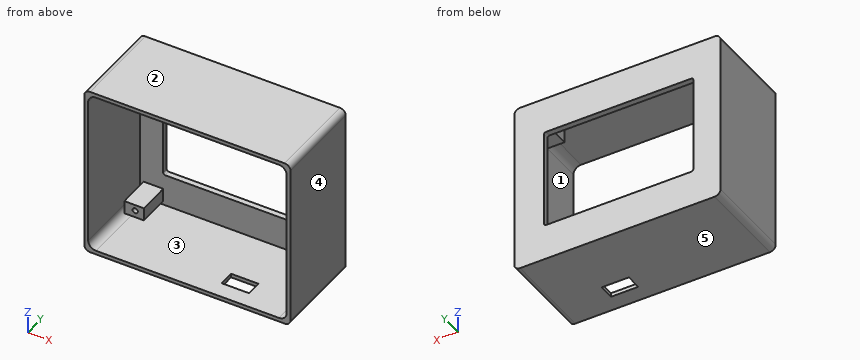
```python
from build123d import *

# Parameters (mm, degrees)
SKETCH1_W           = 106.04
SKETCH1_H           = 88.81
SKETCH1_W_2         = 76.74
SKETCH1_H_2         = 51.6
BOSS_EXTRUDE1_DEPTH = 3
SKETCH1_3_W         = 10
SKETCH1_3_H         = 6.705
SKETCH1_3_R         = 1.35
BOSS_EXTRUDE2_DEPTH = 19.5
SKETCH1_4_W         = 106.04
SKETCH1_4_H         = 88.81
SKETCH1_4_W_2       = 102.04
SKETCH1_4_H_2       = 84.81
BOSS_EXTRUDE3_DEPTH = 47
FILLET1_R           = 4
FILLET2_R           = 3
FILLET3_R           = 1
CUT_EXTRUDE2_REACH  = 115.61
SKETCH3_W           = 14
SKETCH3_H           = 8


with BuildPart() as part:
    # Sketch1 → Boss-Extrude1 (new body)
    with BuildSketch(Plane(origin=(0, 0, 0), x_dir=(1, 0, 0), z_dir=(0, 1, 0))):
        Rectangle(SKETCH1_W, SKETCH1_H)
        with Locations((-0.65, 0)):
            Rectangle(SKETCH1_W_2, SKETCH1_H_2, mode=Mode.SUBTRACT)
    extrude(amount=-BOSS_EXTRUDE1_DEPTH)

    # Sketch1_3 → Boss-Extrude2 (add)
    # profile 1 of 4: a face of its own
    with BuildSketch(Plane(origin=(0, 0, 0), x_dir=(1, 0, 0), z_dir=(0, 1, 0))):
        with Locations((-44.02, -37.0525)):
            Rectangle(SKETCH1_3_W, SKETCH1_3_H)
        with Locations(Location((-43.465, -36.8, 0), (0, 0, 270))):
            Circle(SKETCH1_3_R, mode=Mode.SUBTRACT)
    # profile 2 of 4: a face of its own
    with BuildSketch(Plane(origin=(0, 0, 0), x_dir=(1, 0, 0), z_dir=(0, 1, 0))):
        with Locations((44.02, -37.0525)):
            Rectangle(SKETCH1_3_W, SKETCH1_3_H)
        with Locations(Location((43.465, -36.8, 0), (0, 0, 270))):
            Circle(SKETCH1_3_R, mode=Mode.SUBTRACT)
    # profile 3 of 4: a face of its own
    with BuildSketch(Plane(origin=(0, 0, 0), x_dir=(1, 0, 0), z_dir=(0, 1, 0))):
        with Locations((44.02, 37.0525)):
            Rectangle(SKETCH1_3_W, SKETCH1_3_H)
        with Locations(Location((43.465, 36.8, 0), (0, 0, 270))):
            Circle(SKETCH1_3_R, mode=Mode.SUBTRACT)
    # profile 4 of 4: a face of its own
    with BuildSketch(Plane(origin=(0, 0, 0), x_dir=(1, 0, 0), z_dir=(0, 1, 0))):
        with Locations((-44.02, 37.0525)):
            Rectangle(SKETCH1_3_W, SKETCH1_3_H)
        with Locations(Location((-43.465, 36.8, 0), (0, 0, 270))):
            Circle(SKETCH1_3_R, mode=Mode.SUBTRACT)
    extrude(amount=-BOSS_EXTRUDE2_DEPTH)

    # Sketch1_4 → Boss-Extrude3 (add)
    with BuildSketch(Plane(origin=(0, 0, 0), x_dir=(1, 0, 0), z_dir=(0, 1, 0))):
        Rectangle(SKETCH1_4_W, SKETCH1_4_H)
        Rectangle(SKETCH1_4_W_2, SKETCH1_4_H_2, mode=Mode.SUBTRACT)
    extrude(amount=-BOSS_EXTRUDE3_DEPTH)

    # Fillet1
    fillet1_edges = [part.edges().sort_by_distance(p)[0] for p in [
        (51.02, -25, -42.405),
        (-51.02, -25, -42.405),
        (-51.02, -25, 42.405),
        (51.02, -25, 42.405),
    ]]
    fillet(fillet1_edges, radius=FILLET1_R)

    # Fillet2
    fillet2_edges = [part.edges().sort_by_distance(p)[0] for p in [
        (53.02, -23.5, -44.405),
        (-53.02, -23.5, -44.405),
        (-53.02, -23.5, 44.405),
        (53.02, -23.5, 44.405),
    ]]
    fillet(fillet2_edges, radius=FILLET2_R)

    # Fillet3
    fillet3_edges = [part.edges().sort_by_distance(p)[0] for p in [
        (-39.02, -1.5, 25.8),
        (-39.02, -1.5, -25.8),
        (37.72, -1.5, -25.8),
        (37.72, -1.5, 25.8),
    ]]
    fillet(fillet3_edges, radius=FILLET3_R)

    # Sketch3 → Cut-Extrude2 (cut, up to next)
    with BuildSketch(Plane(origin=(0, 0, -44.405), x_dir=(-1, 0, 0), z_dir=(0, 0, -1)), mode=Mode.PRIVATE) as cut_extrude2_sk1:
        with Locations((-19.52, -34.5)):
            Rectangle(SKETCH3_W, SKETCH3_H)
    cut_extrude2_tool1 = extrude(cut_extrude2_sk1.sketch, amount=-CUT_EXTRUDE2_REACH, mode=Mode.PRIVATE) & part.part
    add(cut_extrude2_tool1.solids().sort_by_distance((19.52, -34.5, -44.405))[0], mode=Mode.SUBTRACT)


solid = part.part
```
CAD build for the part. Positions are in the model's coordinates, mm. Face numbers are marked on the shaded views. A direction names the side the tool comes from. Give positions to 0.01 mm unless a question says otherwise; leave off trailing zeros. Write each loop counter-clockwise with the first axis right and the second up, starting at its lowest first coordinate (ties: lowest second). Pieces come first, ordered by that corner, then holes. Notation, with made-up numbers: (73, 4) -> (132, 4) arc R11 ccw to (132, 19) -> close; hole circle Ø8 at (55, -27). An arc over 180 degrees is marked (long way). Write each question's results on one line, items separated by ' | '.
1. Which spindle directions (+Z, -Z, +X, -X, +Y, -Y) get a long thin tool onto all of the face, cutting with end or side? Do the marked faces 1 and 2. Say none if no direction does.
Geometry check:
face 1: -Y | face 2: +Z, +X, -X, +Y, -Y
2. Drop flat-ended pins along their axis: P1, Ø1, axis at x = 22, z = -43.5, coming from the +Y side; P2, Ø3.5, axis at x = 43, z = -38, coming from the -Y side; P3, Ø1.4, axis at x = -43.5, z = 36.5, coming from the -Y side; P4, Ø1.5, axis at x = 26, z = -24.5, coming from the -Y side. Give the stop position or say it passes through.
Geometry check:
P1: y = 0 | P2: y = -19.5 | P3: y = -3 | P4: through
3. Two-plate mould, pull along Z, no slides. Class the marked faces 3, 4 and 5: pulls with the +Z half, pulls with the -Z half, needs draft (parallel to the pull), parting line crosses it, or undercut.
Geometry check:
face 3: undercut | face 4: needs draft | face 5: pulls with the -Z half
4. Cut at C-C, the plane y = -34. Write the cut outline in (x, z) (3 decimals), then the cut area to 3 significant figures.
Geometry check:
outline: (-53.02, -41.405) arc R3 ccw to (-50.02, -44.405) -> (12.52, -44.405) -> (12.52, -42.405) -> (-47.02, -42.405) arc R4 cw to (-51.02, -38.405) -> (-51.02, 38.405) arc R4 cw to (-47.02, 42.405) -> (47.02, 42.405) arc R4 cw to (51.02, 38.405) -> (51.02, -38.405) arc R4 cw to (47.02, -42.405) -> (26.52, -42.405) -> (26.52, -44.405) -> (50.02, -44.405) arc R3 ccw to (53.02, -41.405) -> (53.02, 41.405) arc R3 ccw to (50.02, 44.405) -> (-50.02, 44.405) arc R3 ccw to (-53.02, 41.405) -> close | area: 741 mm²
5. Cut at D-D, the plane z = -36.8. Write the cut outline in (x, y) (3 decimals).
Geometry check:
outline: (-53.02, -47) -> (-51.02, -47) -> (-51.02, -3) -> (-49.02, -3) -> (-49.02, -19.5) -> (-44.815, -19.5) -> (-44.815, -3) -> (-42.115, -3) -> (-42.115, -19.5) -> (-39.02, -19.5) -> (-39.02, -3) -> (39.02, -3) -> (39.02, -19.5) -> (42.115, -19.5) -> (42.115, -3) -> (44.815, -3) -> (44.815, -19.5) -> (49.02, -19.5) -> (49.02, -3) -> (51.02, -3) -> (51.02, -47) -> (53.02, -47) -> (53.02, 0) -> (-53.02, 0) -> close
6. Cut at A-A, the plane x = -32.5. Write the cut outline in (y, z) (3 decimals).
Geometry check:
outline: (-47, -44.405) -> (0, -44.405) -> (0, -25.8) -> (-3, -25.8) -> (-3, -42.405) -> (-47, -42.405) -> close; (-47, 42.405) -> (-3, 42.405) -> (-3, 25.8) -> (0, 25.8) -> (0, 44.405) -> (-47, 44.405) -> close
7. Cut at B-B, the plane z = -14. Write the cut outline in (x, y), then the cut area to 3 significant figures.
Geometry check:
outline: (-53.02, -47) -> (-51.02, -47) -> (-51.02, -3) -> (-39.02, -3) -> (-39.02, 0) -> (-53.02, 0) -> close; (37.72, -3) -> (51.02, -3) -> (51.02, -47) -> (53.02, -47) -> (53.02, 0) -> (37.72, 0) -> close | area: 264 mm²
8. Wall check: probe 1 along X at (y, z) = (-12, -36.8) (3 decimals); probe 2 along Z at (x, y) = (-41, -8) (3 decimals); probe 3 along X at (y, z) = (-28, -2.5). Give the ranges that are in metal, low to high. Write a range as [from, to].
Geometry check:
probe 1: [-53.02, -51.02], [-49.02, -44.815], [-42.115, -39.02], [39.02, 42.115], [44.815, 49.02], [51.02, 53.02] | probe 2: [-44.405, -42.405], [-40.405, -33.7], [33.7, 40.405], [42.405, 44.405] | probe 3: [-53.02, -51.02], [51.02, 53.02]
